from build123d import *

# Parameters (mm, degrees)
SKETCH1_W           = 19.05
SKETCH1_H           = 19.05
BOSS_EXTRUDE2_DEPTH = 6.35
SKETCH8_W           = 217.17
SKETCH8_H           = 38.1
BOSS_EXTRUDE4_DEPTH = 6.35
SKETCH8_5_W         = 217.17
SKETCH8_5_H         = 38.1
BOSS_EXTRUDE5_DEPTH = 6.4262
SKETCH9_W           = 19.05
SKETCH9_H           = 38.1
LPATTERN3_COUNT     = 11
LPATTERN3_PITCH     = 19.812
SKETCH15_R          = 12.192
BOSS_EXTRUDE6_DEPTH = 6.35
SKETCH16_W          = 38.1
SKETCH16_H          = 22.073264639
CUT_EXTRUDE1_DEPTH  = 3.302


with BuildPart() as part:
    # Sketch1 → Boss-Extrude2 (new body)
    with BuildSketch(Plane(origin=(0, 0, 0), x_dir=(1, 0, 0), z_dir=(0, 1, 0))):
        with Locations((9.525, -9.525)):
            Rectangle(SKETCH1_W, SKETCH1_H)
    extrude(amount=BOSS_EXTRUDE2_DEPTH)

    # Sketch8 → Boss-Extrude4 (add)
    with BuildSketch(Plane(origin=(0, 0, 0), x_dir=(1, 0, 0), z_dir=(0, 1, 0))):
        with Locations((108.585, -9.525)):
            Rectangle(SKETCH8_W, SKETCH8_H)
    extrude(amount=BOSS_EXTRUDE4_DEPTH)

    # Sketch8_5 → Boss-Extrude5 (add)
    with BuildSketch(Plane(origin=(0, 0, 0), x_dir=(1, 0, 0), z_dir=(0, 1, 0))):
        with Locations((108.585, -9.525)):
            Rectangle(SKETCH8_5_W, SKETCH8_5_H)
    extrude(amount=-BOSS_EXTRUDE5_DEPTH)

    # Sketch9 → Loft3 section 0
    with BuildSketch(Plane(origin=(0, 6.35, 0), x_dir=(1, 0, 0), z_dir=(0, 1, 0)), mode=Mode.PRIVATE) as loft3_s0:
        with Locations((9.525, -9.525)):
            Rectangle(SKETCH9_W, SKETCH9_H)
    loft3 = loft([loft3_s0.sketch, Vertex(9.525, 26.0731, 19.05)])

    # LPattern3: Loft3 ×11
    with Locations(*[(i * LPATTERN3_PITCH, 0, 0) for i in range(1, LPATTERN3_COUNT)]):
        add(loft3)

    # Sketch15 → Boss-Extrude6 (add)
    with BuildSketch(Plane.XZ.offset(6.4262)):
        with Locations((179.07, 9.525)):
            Circle(SKETCH15_R)
        with Locations((38.1, 9.525)):
            Circle(SKETCH15_R)
        with Locations((108.585, 9.525)):
            Circle(SKETCH15_R)
    extrude(amount=BOSS_EXTRUDE6_DEPTH)

    # Sketch16 → Cut-Extrude1 (cut)
    with BuildSketch(Plane(origin=(219.71, 0, 0), x_dir=(0, 0, -1), z_dir=(1, 0, 0))):
        with Locations((-9.525, 4.61043232)):
            Rectangle(SKETCH16_W, SKETCH16_H)
    extrude(amount=-CUT_EXTRUDE1_DEPTH, mode=Mode.SUBTRACT)


solid = part.part
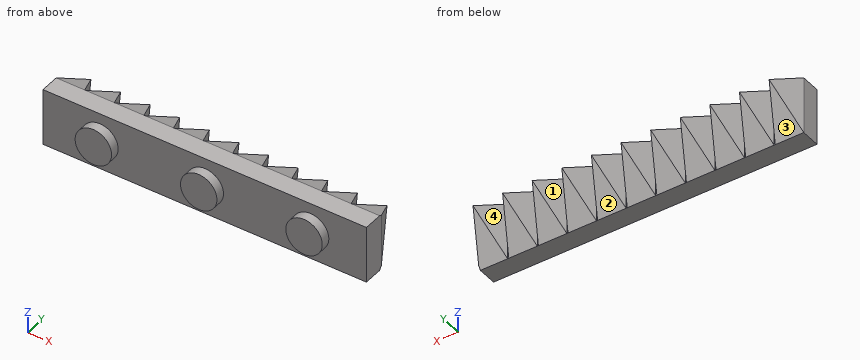
Here's how the part is built. I have some questions about the finished solid (model axes, mm). Face numbers are marked on the shaded views. A direction names the side the tool comes from. Give positions to 0.01 mm unless a question says otherwise; leave off trailing zeros. Order: outer loops, then holes, each group sorted by start corner. A loop starts at its lowest first (then second) coordinate and runs counter-clockwise, first axis right, second up. Notation, with made-up numbers: M 12,40 L 27,40 A31 cw 27,75 Z; hole C -40,-32 d6. An arc over 180 degrees is marked long. Answer as a JSON object with one key per item and string values. Group by question number.
1) I'm going to push flat-ended pins straight in: pin 1 Ø3 at (x, y) = (182.5, 15) entering from +Z; pin 2 Ø8 at (x, z) = (54, 16) entering from +Y; pin 3 Ø11.5 at (x, z) = (140, 16.5) entering from -Y; pin 4 Ø1.5 at (x, y) = (139.5, 13) entering from +Z. Where does each tip first touch, or does it pass through?
2) Suppose I cut it at A-A, the plane x = 171. Write out the boundary of the cut face in (y, z) (3 decimals).
3) On a 3-axis mill with a long thin cutter (end or side, diameter ignored), from which of +Z, -Z, +X, -X, +Y, -Y can I reach the whole of each face in a straight line? I mean the marked faces 3 and 4. Say none if no direction works.
4) Suppose I cut it at B-B, the plane y = 23.5. Count the separate pieces of the cut face and the enclosed holes in it, plus the area to 3 significant figures.
5) Please list where these lines run through material, in increasing order: L1, parallel to X at y = -7, z = 16; L2, parallel to Y at x = 110, z = 10; L3, parallel to X at y = -10.5, z = 19.5. Write a range as [from, to].
6) We'd pull the mould along X, two halves only. Please class the marked faces 1 and 2: pulls with the +X half, pulls with the -X half, needs draft (parallel to the pull), parting line crosses it, or undercut.
Results found:
{
 "1": {"pin 1": "z = 25.12", "pin 2": "y = 24.26", "pin 3": "y = -6.43", "pin 4": "through"},
 "2": {"outline": "M -12.776,0.386 L -6.426,0.386 L -6.426,-9.525 L 6.35,-9.525 L 19.905,10.113 L 19.905,22.029 L 6.35,28.575 L -6.426,28.575 L -6.426,18.664 L -12.776,18.664 Z"},
 "3": {"face 3": "-Z, +X, -X, +Y", "face 4": "+Z, -Z, +Y"},
 "4": {"separate pieces": "11", "enclosed holes": "0", "area": "136 mm²"},
 "5": {"L1": "[27.77, 48.43], [98.25, 118.92], [168.74, 189.4]", "L2": "[-12.78, 19.83]", "L3": "[31.09, 45.11], [101.57, 115.6], [172.06, 186.08]"},
 "6": {"face 1": "undercut", "face 2": "needs draft"}
}
